```python
from build123d import *

# Parameters (mm, degrees)
CUT_EXTRUDE2_DEPTH      = 115.535519609
CUT_EXTRUDE2_DEPTH_BACK = 115.535519609
SKETCH2_R               = 25
SKETCH3_R               = 50
CUT_EXTRUDE4_DEPTH      = 11


with BuildPart() as part:
    # Sketch1 → Revolve1 (revolve)
    with BuildSketch(Plane.XY, mode=Mode.PRIVATE) as revolve1_sk:
        Polygon((-63.203744258, 71.61674857), (-63.203744258, 41.61674857), (-59.626173828, 41.61674857), (-59.626173828, 38.61674857), (-63.203744258, 38.61674857), (-63.203744258, 33.61674857), (-59.626173828, 33.61674857), (-59.626173828, 30.61674857), (-63.203744258, 30.61674857), (-63.203744258, 25.61674857), (-59.626173828, 25.61674857), (-59.626173828, 22.61674857), (-63.203744258, 22.61674857), (-63.203744258, 17.61674857), (-59.626173828, 17.61674857), (-59.626173828, 14.61674857), (-63.203744258, 14.61674857), (-63.203744258, -64.740949558), (0, -64.740949558), (0, -57.740949558), (-53.203744258, -57.740949558), (-53.203744258, 56.61674857), (0, 56.61674857), (0, 66.852401658), (-41.78964032, 66.852401658), (-53.203744258, 71.61674857), align=None)
    revolve(revolve1_sk.sketch.rotate(Axis((0, 112.693468535, 0), (0, -1, 0)), 270), axis=Axis((0, 112.693468535, 0), (0, -1, 0)))

    # Sketch2 → Cut-Extrude2 (cut, two sides: drawn at the far end of the back side and taken through both)
    with BuildSketch(Plane.XY.offset(-CUT_EXTRUDE2_DEPTH_BACK)):
        with Locations((0, -25.062100494)):
            Circle(SKETCH2_R)
    extrude(amount=CUT_EXTRUDE2_DEPTH + CUT_EXTRUDE2_DEPTH_BACK, mode=Mode.SUBTRACT)

    # Sketch3 → Cut-Extrude4 (cut)
    with BuildSketch(Plane.XZ.offset(64.740949558)):
        with Locations(Location((0, 0, 0), (0, 0, 270))):
            Circle(SKETCH3_R)
    extrude(amount=-CUT_EXTRUDE4_DEPTH, mode=Mode.SUBTRACT)


solid = part.part
```
Geometry: final body of the model. Coordinates: model frame, mm. A direction names the side the tool comes from. Give positions to 0.01 mm unless a question says otherwise; leave off trailing zeros. Loops run counter-clockwise (first coordinate to the right, second up) from the corner with the lowest first, then second, coordinate; pieces in that order, holes last. Notation, with made-up numbers: (-2, 69.5) -> (16, 69.5) arc R9 cw to (16, 83.5) -> close; hole circle Ø1 at (86.25, 33.5). An arc over 180 degrees is marked (long way). Use CSV: the item, a comma, the result in double quotes.
(1) Cut plane A-A (x = 0). Count the separate pieces of the cut face and the enclosed holes in it, plus the area to 3 significant figures.
From the geometry:
separate pieces,"3"
enclosed holes,"0"
area,"2,830 mm^2"
(2) Pull-direction query (Z, two-part tool) for faces 1 (the face through (47, 17.617, -38)), 2 (the face through (-1, 66.852, 1)), 3 (the face through (-50.28, 16.1, 32.05)); classes: released by +Z, released by -Z, zero draft, split by the parting line, or undercut.
From the geometry:
face 1,"zero draft"
face 2,"undercut"
face 3,"split by the parting line"
(3) Cut plane B-B (y = -52). Output: boundary loops of the cut face in (x, z), plus the area to 3 significant figures.
From the geometry:
outline,"circle Ø126.41 at (0, 0); hole circle Ø106.41 at (0, 0)"
area,"3,660 mm^2"
(4) First-contact query: P1, Ø5, axis at x = -35.5, y = 9, coming from the -Z side; P2, Ø1, axis at x = -18.5, y = -10, coming from the +Z side; P3, Ø1.5, axis at x = 13, y = 49.5, coming from the -Z side; P4, Ø5, axis at x = 18, z = 8, coming from the -Y side. Flat tips, straight axial feed; report the tip coordinate or a pass-through.
From the geometry:
P1,"z = -53.9"
P2,"through"
P3,"z = -62.01"
P4,"y = 56.62"
(5) Ray query, line 1 along X through (y, z) = (19, 1); line 2 along Y through (x, z) = (0, -56); line 3 along X through (y, z) = (39.5, -8). Return the intervals inside material, ascending. Write a range as [from, to].
From the geometry:
line 1,"[-63.2, -53.19], [53.19, 63.2]"
line 2,"[-64.74, -50.06], [-0.06, 71.62]"
line 3,"[-59.09, -52.6], [52.6, 59.09]"
(6) Access query for faces 4 (the face through (-24.976, -23.963, 54.97)), 5 (the face through (15.02, -61.29, -47.69)), 6 (the face through (-2.339, 0.238, -53.152)). Directions: +Z, -Z, +X, -X, +Y, -Y. A direction counts if a zero-diameter tool reaches every point of the face in a straight line with its end or side. Return the directions, or none.
From the geometry:
face 4,"+Z, -Z"
face 5,"-Y"
face 6,"none"
